Read the model definition and answer for the solid it produces. Units are mm, in the model's axes. Give positions to 0.01 mm unless a question says otherwise; leave off trailing zeros. Order: outer loops, then holes, each group sorted by start corner. A loop starts at its lowest first (then second) coordinate and runs counter-clockwise, first axis right, second up. Notation, with made-up numbers: M -40,83.5 L 2,83.5 A18 cw 2,113.5 Z; hole C -31,4.5 d7. An arc over 180 degrees is marked long. One line per item, written item: value. Start each with the question number.
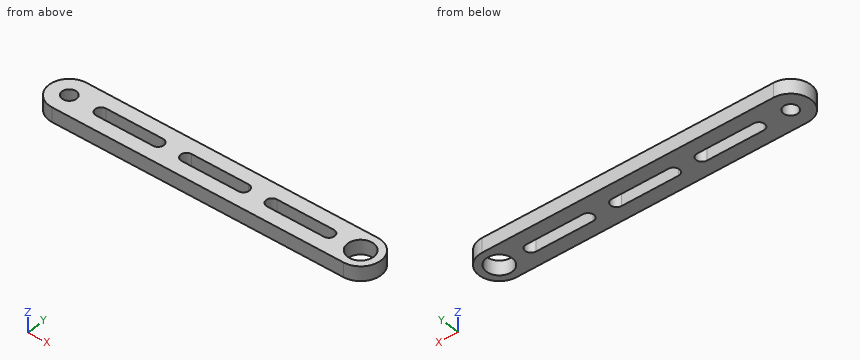
from build123d import *

# Parameters (mm, degrees)
SKETCH_2_R                 = 4.5
EXTRUDE_1_DEPTH            = 2.5
CUT_EXTRUDE_1_DEPTH        = 10
PATTERN_LINEAR_1_COUNT     = 2
PATTERN_LINEAR_1_PITCH     = 30
PATTERN_LINEAR_1_COL_COUNT = 2
PATTERN_LINEAR_1_COL_PITCH = 30
EXTRUDE_START              = -5
SKETCH_5_R                 = 4.5
SKETCH_5_R_2               = 2.5
EXTRUDE_3_DEPTH            = 5


with BuildPart() as part:
    # 草图2 → 凸台-拉伸1 (new, symmetric)
    with BuildSketch(Plane.XY):
        with BuildLine():
            Line((-51.175, 7), (51.175, 7))
            ThreePointArc((51.175, 7), (58.175, 0), (51.175, -7))
            Line((51.175, -7), (-51.175, -7))
            ThreePointArc((-51.175, -7), (-58.175, 0), (-51.175, 7))
        make_face()
        with Locations((51.175, 0)):
            Circle(SKETCH_2_R, mode=Mode.SUBTRACT)
        with Locations((-51.175, 0)):
            Circle(SKETCH_2_R, mode=Mode.SUBTRACT)
    extrude(amount=EXTRUDE_1_DEPTH, both=True)

    # 草图3 → 切除-拉伸1 (cut)
    with BuildSketch(Plane.XY.offset(2.5)):
        with BuildLine():
            Line((-10, 2), (10, 2))
            ThreePointArc((10, 2), (12, 0), (10, -2))
            Line((10, -2), (-10, -2))
            ThreePointArc((-10, -2), (-12, 0), (-10, 2))
        make_face()
    cut_extrude_1 = extrude(amount=-CUT_EXTRUDE_1_DEPTH, mode=Mode.SUBTRACT)

    # 阵列(线性)1: 切除-拉伸1 ×2
    with Locations(*[(-i * PATTERN_LINEAR_1_PITCH, 0, 0) for i in range(1, PATTERN_LINEAR_1_COUNT)]):
        add(cut_extrude_1, mode=Mode.SUBTRACT)

    # 阵列(线性)1 col: 切除-拉伸1 ×2
    with Locations(*[(i * PATTERN_LINEAR_1_COL_PITCH, 0, 0) for i in range(1, PATTERN_LINEAR_1_COL_COUNT)]):
        add(cut_extrude_1, mode=Mode.SUBTRACT)

    # 草图5 → 凸台-拉伸3 (add)
    with BuildSketch(Plane.XY.offset(2.5).offset(EXTRUDE_START)):
        with Locations((-51.175, 0)):
            Circle(SKETCH_5_R)
        with Locations((-51.175, 0)):
            Circle(SKETCH_5_R_2, mode=Mode.SUBTRACT)
    extrude(amount=EXTRUDE_3_DEPTH)


solid = part.part
Q1. Find section B-B, the plane z = -0.2. Give the vertices of the cut face in (x, y) (3 decimals).
Q2. Find section A-A, the plane y = 0. Give the vertices of the cut face in (x, z) (3 decimals).
Q3. Find section C-C, the plane x = 29.5. Give the vertices of the cut face in (y, z).
Q4. Consider probe 1 along Y at (x, z) = (20, 0.25); probe 2 along X at (y, z) = (1.25, -0.45); probe 3 along X at (y, z) = (-1, 0.2). Determine where each line is inside the solid, lowest interval first.
Q5. Each of these flat-tipped pins is pushed along its axis until it touches: pin 1 (8 mm diameter, centred on x = 24, y = -1, fed in from +Z); pin 2 (2 mm diameter, centred on y = 5, z = 1, fed in from -X); pin 3 (3 mm diameter, centred on y = -3.5, z = 0, fed in from -X). Where does it stop, or does it pass through?
Evaluation:
1. outline: M -51.175,-7 L 51.175,-7 A7 ccw 51.175,7 L -51.175,7 A7 ccw Z; hole C -51.175,0 d5; hole M -40,-2 L -20,-2 A2 ccw -20,2 L -40,2 A2 ccw Z; hole M -10,-2 L 10,-2 A2 ccw 10,2 L -10,2 A2 ccw Z; hole M 20,-2 L 40,-2 A2 ccw 40,2 L 20,2 A2 ccw Z; hole C 51.175,0 d9
2. outline: M -58.175,-2.5 L -53.675,-2.5 L -53.675,2.5 L -58.175,2.5 Z; M -48.675,-2.5 L -42,-2.5 L -42,2.5 L -48.675,2.5 Z; M -18,-2.5 L -12,-2.5 L -12,2.5 L -18,2.5 Z; M 12,-2.5 L 18,-2.5 L 18,2.5 L 12,2.5 Z; M 42,-2.5 L 46.675,-2.5 L 46.675,2.5 L 42,2.5 Z; M 55.675,-2.5 L 58.175,-2.5 L 58.175,2.5 L 55.675,2.5 Z
3. outline: M -7,-2.5 L -2,-2.5 L -2,2.5 L -7,2.5 Z; M 2,-2.5 L 7,-2.5 L 7,2.5 L 2,2.5 Z
4. probe 1: -7 to -2, 2 to 7
4. probe 2: -58.06 to -53.34, -49.01 to -41.56, -18.44 to -11.56, 11.56 to 18.44, 41.56 to 46.85, 55.5 to 58.06
4. probe 3: -58.1 to -53.47, -48.88 to -41.73, -18.27 to -11.73, 11.73 to 18.27, 41.73 to 46.79, 55.56 to 58.1
5. pin 1: z = 2.5
5. pin 2: x = -56.92
5. pin 3: x = -57.88
